Verification items for the finished model (mm, model axes). A direction names the side the tool comes from. Give positions to 0.01 mm unless a question says otherwise; leave off trailing zeros. Write each loop counter-clockwise with the first axis right and the second up, starting at its lowest first coordinate (ties: lowest second). Pieces come first, ordered by that corner, then holes. Notation, with made-up numbers: (32.5, -7.5) - (53.5, -7.5) arc R19 ccw to (53.5, 29.5) - close; hole circle Ø9 at (84, -20). An arc over 180 degrees is marked (long way). Answer as a JSON object with one key per item and string values. Group by question number.
Item 1: Draft check along Z on faces 1 (the face through (83.235, 23.533, 45.505)), 2 (the face through (100, 0, 1)), 3 (the face through (26, 130, 26)). Enter one of: +Z half, -Z half, draft (parallel to the pull), parting line (faces both ways), or undercut.
Item 2: Go/stop test with flat-tipped pins: pin 1 (2 mm diameter, centred on y = 129.5, z = -3.5, fed in from +X); pin 2 (20 mm diameter, centred on x = 111.5, z = 15.5, fed in from +Y); pin 3 (2 mm diameter, centred on x = 50, y = 64, fed in from -Z). Record where each tip stops, or that it passes through.
Item 3: Scan lines: line 1 along X through (y, z) = (141, 0); line 2 along X through (y, z) = (17.5, 0); line 3 along X through (y, z) = (72.5, 2). Record each from-to range of solid material in increasing order. Write a range as [from, to].
Item 4: Sectioned sample at C-C, the plane z = 41. Record the boundary of the cut face in (x, y), and give its area (3 significant figures).
Item 5: Sectioned sample at D-D, the plane y = 135. Record the boundary of the cut face in (x, z), and give its area (3 significant figures).
Item 6: Sectioned sample at A-A, the plane x = 0. Record the boundary of the cut face in (y, z).
Item 7: Sectioned sample at B-B, the plane z = 0. Record the boundary of the cut face in (x, y).
Item 8: Tool access check on faces 4 (the face through (-76.02, 33.43, 4.77)), 5 (the face through (-109, 25, -1)), 6 (the face through (110, 25, 1)). Record the directions out of +Z, -Z, +X, -X, +Y, -Y that give a thin tool (end or side, any length) a straight path to the whole face; none if there is none.
```python
from build123d import *

# Parameters (mm, degrees)
BOSS_EXTRUDE2_DEPTH = 75
SKETCH2_OUTSIDE_W   = 370.368
SKETCH2_OUTSIDE_H   = 220.368
SKETCH2_OUTSIDE_R   = 12.5
CUT_EXTRUDE3_DEPTH  = 150
BOSS_EXTRUDE3_REACH = 227
SKETCH3_R           = 75


with BuildPart() as part:
    # Sketch1 → Boss-Extrude2 (new, symmetric)
    with BuildSketch(Plane.XY):
        with BuildLine():
            Line((150, 25), (83.240615087, 25))
            ThreePointArc((83.240615087, 25), (91.224995055, 12.990386393), (97.488460856, 0))
            Line((97.488460856, 0), (150, 0))
            Line((150, 0), (150, 25))
        make_face()
        with BuildLine():
            Line((-48, 25), (-83.240615087, 25))
            ThreePointArc((-83.240615087, 25), (-91.224995055, 12.990386393), (-97.488460856, 0))
            Line((-97.488460856, 0), (-69.84983894, 0))
            ThreePointArc((-69.84983894, 0), (-60.236169654, 13.646024213), (-48, 25))
        make_face()
        with BuildLine():
            ThreePointArc((97.488460856, 0), (91.224995055, 12.990386393), (83.240615087, 25))
            Line((83.240615087, 25), (48, 25))
            ThreePointArc((48, 25), (60.236169654, 13.646024213), (69.84983894, 0))
            Line((69.84983894, 0), (97.488460856, 0))
        make_face()
        with BuildLine():
            ThreePointArc((83.240615087, 25), (0, 66), (-83.240615087, 25))
            Line((-83.240615087, 25), (-48, 25))
            ThreePointArc((-48, 25), (0, 41), (48, 25))
            Line((48, 25), (83.240615087, 25))
        make_face()
        with BuildLine():
            Line((-48, 25), (-83.240615087, 25))
            ThreePointArc((-83.240615087, 25), (-91.224995055, 12.990386393), (-97.488460856, 0))
            Line((-97.488460856, 0), (-69.84983894, 0))
            ThreePointArc((-69.84983894, 0), (-60.236169654, 13.646024213), (-48, 25))
        make_face()
        with BuildLine():
            ThreePointArc((97.488460856, 0), (91.224995055, 12.990386393), (83.240615087, 25))
            Line((83.240615087, 25), (48, 25))
            ThreePointArc((48, 25), (60.236169654, 13.646024213), (69.84983894, 0))
            Line((69.84983894, 0), (97.488460856, 0))
        make_face()
        with BuildLine():
            Line((-83.240615087, 25), (-150, 25))
            Line((-150, 25), (-150, 0))
            Line((-150, 0), (-97.488460856, 0))
            ThreePointArc((-97.488460856, 0), (-91.224995055, 12.990386393), (-83.240615087, 25))
        make_face()
    extrude(amount=BOSS_EXTRUDE2_DEPTH, both=True)

    # Sketch2 outside → Cut-Extrude3 (cut)
    # profile 1 of 3: a face of its own
    with BuildSketch(Plane(origin=(0, 0, 0), x_dir=(1, 0, 0), z_dir=(0, 1, 0))):
        Rectangle(SKETCH2_OUTSIDE_W, SKETCH2_OUTSIDE_H)
        with BuildLine():
            Line((135, -22.912878475), (30, -68.738635424))
            ThreePointArc((30, -68.738635424), (0, -75), (-30, -68.738635424))
            Line((-30, -68.738635424), (-135, -22.912878475))
            ThreePointArc((-135, -22.912878475), (-150, 0), (-135, 22.912878475))
            Line((-135, 22.912878475), (-30, 68.738635424))
            ThreePointArc((-30, 68.738635424), (0, 75), (30, 68.738635424))
            Line((30, 68.738635424), (135, 22.912878475))
            ThreePointArc((135, 22.912878475), (150, 0), (135, -22.912878475))
        make_face(mode=Mode.SUBTRACT)
    # profile 2 of 3: a face of its own
    with BuildSketch(Plane(origin=(0, 0, 0), x_dir=(1, 0, 0), z_dir=(0, 1, 0))):
        with Locations(Location((125, 0, 0), (0, 0, 180))):
            Circle(SKETCH2_OUTSIDE_R)
    # profile 3 of 3: a face of its own
    with BuildSketch(Plane(origin=(0, 0, 0), x_dir=(1, 0, 0), z_dir=(0, 1, 0))):
        with Locations(Location((-125, 0, 0), (0, 0, 180))):
            Circle(SKETCH2_OUTSIDE_R)
    extrude(amount=CUT_EXTRUDE3_DEPTH, mode=Mode.SUBTRACT)

    # Sketch3 → Boss-Extrude3 (add, up to next)
    with BuildSketch(Plane(origin=(0, 150, 0), x_dir=(1, 0, 0), z_dir=(0, 1, 0)), mode=Mode.PRIVATE) as boss_extrude3_sk1:
        with Locations(Location((0, 0, 0), (0, 0, 113.578178478))):
            Circle(SKETCH3_R)
    boss_extrude3_tool1 = extrude(boss_extrude3_sk1.sketch, amount=-BOSS_EXTRUDE3_REACH, mode=Mode.PRIVATE) - part.part
    add(boss_extrude3_tool1.solids().sort_by_distance((0, 150, 0))[0])

    # Sketch5 → Cut-Revolve3 (revolve, cut)
    with BuildSketch(Plane.XY, mode=Mode.PRIVATE) as cut_revolve3_sk:
        Polygon((0, 150), (60.25406126, 150), (60.25406126, 130), (35, 130), (35, 0), (0, 0), align=None)
    revolve(cut_revolve3_sk.sketch.rotate(Axis((0, 0, 0), (0, -1, 0)), 90), axis=Axis((0, 0, 0), (0, -1, 0)), mode=Mode.SUBTRACT)


solid = part.part
```
Geometry check:
{
 "1": {"face 1": "+Z half", "face 2": "draft", "face 3": "undercut"},
 "2": {"pin 1": "x = 74.96", "pin 2": "y = 25", "pin 3": "z = -56.78"},
 "3": {"line 1": "[-75, -60.25], [60.25, 75]", "line 2": "[-150, -137.5], [-112.5, -56.64], [56.64, 112.5], [137.5, 150]", "line 3": "[-74.97, -34.94], [34.94, 74.97]"},
 "4": {"outline": "(-93.56, 0) - (-69.85, 0) arc R80 cw to (69.85, 0) - (93.56, 0) - (93.56, 25) - (83.24, 25) arc R105 ccw to (62.8, 45.15) - (62.8, 150) - (44.15, 150) - (44.15, 130) - (-44.15, 130) - (-44.15, 150) - (-62.8, 150) - (-62.8, 45.15) arc R105 ccw to (-83.24, 25) - (-93.56, 25) - close", "area": "15,000 mm^2"},
 "5": {"outline": "circle Ø150 at (0, 0); hole circle Ø120.51 at (0, 0)", "area": "6,270 mm^2"},
 "6": {"outline": "(41, -75) - (150, -75) - (150, -60.25) - (130, -60.25) - (130, -35) - (41, -35) - close; (41, 35) - (130, 35) - (130, 60.25) - (150, 60.25) - (150, 75) - (41, 75) - close"},
 "7": {"outline": "(-150, 0) - (-137.5, 0) - (-137.5, 25) - (-150, 25) - close; (-112.5, 0) - (-69.85, 0) arc R80 cw to (-35, 32.94) - (-35, 130) - (-60.25, 130) - (-60.25, 150) - (-75, 150) - (-75, 34.48) arc R105 ccw to (-83.24, 25) - (-112.5, 25) - close; (35, 32.94) arc R80 cw to (69.85, 0) - (112.5, 0) - (112.5, 25) - (83.24, 25) arc R105 ccw to (75, 34.48) - (75, 150) - (60.25, 150) - (60.25, 130) - (35, 130) - close; (137.5, 0) - (150, 0) - (150, 25) - (137.5, 25) - close"},
 "8": {"face 4": "-X, +Y", "face 5": "+Z, -Z, -X, +Y", "face 6": "+Z, -Z, +X, +Y"}
}
